Autodesk Inventor part; units mm, degrees
ref_plane "YZ Plane" through (0, 0, 0) normal (1, 0, 0) x (0, 1, 0)
ref_plane "XZ Plane" through (0, 0, 0) normal (0, 1, 0) x (-1, 0, 0)
ref_plane "XY Plane" through (0, 0, 0) normal (0, 0, 1) x (1, 0, 0)
sketch "スケッチ1" plane through (0, 0, 0) normal (1, 0, 0) x (0, 1, 0)
  circle A0 centre (0, 0) radius 120
  circle A1 centre (0, 0) radius 130
  line L0 (0, 0) -> (84.8528, 84.8528)
  line L1 (0, 0) -> (0, 120)
  line L2 (84.8528, 84.8528) -> (91.9239, 91.9239)
  line L3 (-130, 237.6299) -> (-130, -340.0687)
  line L4 (58.9191, 140) -> (-130, 140)
  line L5 (0, 0) -> (-130, 0)
  line L6 (0, 120) -> (0, 130)
  line L7 (-120, 140) -> (-120, 130)
  line L8 (-120, 130) -> (0, 130)
  line L9 (-120, 0) -> (-120, 140)
  line L10 (-110, 140) -> (-110, 130)
  point P0 (-120, 0)
  dimension "d0" = 240
  dimension "d1" = 10
  dimension "d2" = 45
  dimension "d3" = 140
  dimension "d4" = 0
  dimension "d5" = 10
  dimension "d6" = 10
  dimension "d8" = 10
revolve "回転1" add sketch "スケッチ1" angle 80 about axis through (0, 0, 0) along (0, 1, 0) contours L9 A1 L6 A0 | L9 L8 A1 | L7 L4 L10 L8
sketch "スケッチ2" plane through (0, -110, 140) normal (0, 1, 0) x (1, 0, 0)
  line L0 (137.8731, 115.6893) -> (0, 140)
  line L1 (0, 0) -> (0, 140)
  circle A0 centre (0, 140) radius 140
  circle A1 centre (0, 140) radius 135
  point P0 (46.1727, 13.1415)
  point P1 (116.9134, 72.5)
  dimension "d9" = 5
  dimension "d10" = 20
  dimension "d11" = 20
hole "穴1" at (46.1727, -110, 126.8585) at (116.9134, -110, 67.5) direction (0, -1, 0) diameter 3.4 end through all
sketch "スケッチ3" plane through (0, -120, 0) normal (0, -1, 0) x (1, 0, 0)
  line L0 (17, -30) -> (-17, -30)
  line L1 (-17, -30) -> (-17, 30)
  line L2 (-17, 30) -> (17, 30)
  line L3 (17, 30) -> (17, -30)
  circle A0 centre (14.5, 7.5) radius 4
  point P0 (0, 0)
  point P1 (17, 10.6225)
  point P2 (17, 4.3775)
  dimension "d19" = 34
  dimension "d20" = 60
  dimension "d21" = 30
  dimension "d22" = 17
  dimension "d25" = 8
  dimension "d26" = 2.5
  dimension "d27" = 22.5
extrude "押し出し1" cut sketch "スケッチ3" against normal blind 10
fillet "フィレット2" radius 2 5 edges at (17, -119.376, 2.9976) (17, -119.3545, 4.3775) (17, -119.1569, 10.6225) (17, -117.4696, 30) (0, -118.0948, 30)
properties part number "belt_liner_v1_3DP_C_B_U" material "ABS プラスチック"
Here's how the part is built. I have some questions about the finished solid (model axes, mm). A direction names the side the tool comes from. Give positions to 0.01 mm unless a question says otherwise; leave off trailing zeros. Order: outer loops, then holes, each group sorted by start corner. A loop starts at its lowest first (then second) coordinate and runs counter-clockwise, first axis right, second up. Notation, with made-up numbers: M 25.5,33 L 70.5,33 A21 cw 70.5,47 Z; hole C 45,83 d9. An arc over 180 degrees is marked long. Answer as a JSON object with one key per item and string values. Group by question number.
1) Suppose I cut it at D-D, the plane y = -27.5. Write out the boundary of the cut face in (x, z) (3 decimals).
2) I'm going to push flat-ended pins straight in: pin 1 Ø12 at (x, y) = (93.5, -18.5) entering from -Z; pin 2 Ø6 at (y, z) = (-15.5, 121) entering from +X; pin 3 Ø1.5 at (x, y) = (37.5, -20) entering from +Z; pin 4 Ø3 at (x, z) = (46.17, 126.86) entering from +Y. Where does each tip first touch, or does it pass through?
3) Please list where these lines run through material, in increasing order: L1, parallel to Y at x = 106, z = 85; L2, parallel to X at y = -116.5, z = 67.5; L3, parallel to X at y = -113, z = 67. Write a range as [from, to].
4) Suppose I cut it at A-A, the plane x = 101.5. Write out the boundary of the cut face in (y, z), plus the area to 3 significant figures.
5) On a 3-axis mill with a long thin cutter (end or side, diameter ignored), from which of +Z, -Z, +X, -X, +Y, -Y can I reach the whole of each face in a straight line? I mean faces 1 (the flat face through (17, -118, 22)), 2 (the flat face through (85, -110, 103)), 3 (the flat face through (105.55, -82.5, 18.61)). Say none if no direction works.
6) Suppose I cut it at C-C, the plane y = -69.5. Write out the boundary of the cut face in (x, z) (3 decimals).
7) Suppose I cut it at B-B, the plane z = 85. Write out the boundary of the cut face in (x, y).
Results found:
{
 "1": {"outline": "M 0,116.806 A116.806 cw 115.032,20.283 L 128.025,22.574 A130 ccw 0,130 Z"},
 "2": {"pin 1": "z = 64.31", "pin 2": "x = 54.55", "pin 3": "z = 124.7", "pin 4": "through"},
 "3": {"L1": "[-120, -110]", "L2": "[0, 115.21], [118.61, 122.65]", "L3": "[0, 115.29], [118.54, 122.93]"},
 "4": {"outline": "M -120,17.9 L -61.46,17.9 A64.01 cw 0,64.01 L 0,81.23 L -110,81.23 L -110,96.42 L -120,96.42 Z", "area": "5,660 mm²"},
 "5": {"face 1": "-Z, -X, +Y, -Y", "face 2": "+Z, +X, +Y", "face 3": "-Z, +X, +Y, -Y"},
 "6": {"outline": "M 0,97.825 A97.825 cw 96.339,16.987 L 128.025,22.574 A130 ccw 0,130 Z"},
 "7": {"outline": "M 0,-120 L 111.24,-120 L 111.24,-110 L 98.36,-110 L 98.36,0 L 84.71,0 A84.71 cw 0,-84.71 Z"}
}
